from build123d import *

# Parameters (mm, degrees)
SKETCH1_R           = 11.025
BOSS_EXTRUDE1_DEPTH = 10
SKETCH3_R           = 11.025
SKETCH3_R_2         = 6
BOSS_EXTRUDE2_DEPTH = 4
FILLET1_R           = 4
FILLET2_R           = 1
CUT_EXTRUDE1_REACH  = 12
SKETCH4_R           = 2.6


with BuildPart() as part:
    # Sketch1 → Boss-Extrude1 (new body)
    with BuildSketch(Plane(origin=(0, 0, 0), x_dir=(1, 0, 0), z_dir=(0, 1, 0))):
        with BuildLine():
            Line((-40, -16.45412), (40, -16.45412))
            Line((40, -16.45412), (40, 0))
            Line((40, 0), (20.55, 0))
            ThreePointArc((20.55, 0), (0, 20.55), (-20.55, 0))
            Line((-20.55, 0), (-40, 0))
            Line((-40, 0), (-40, -16.45412))
        make_face()
        Circle(SKETCH1_R, mode=Mode.SUBTRACT)
    extrude(amount=BOSS_EXTRUDE1_DEPTH)

    # Sketch3 → Boss-Extrude2 (add)
    with BuildSketch(Plane.XZ):
        Circle(SKETCH3_R)
        Circle(SKETCH3_R_2, mode=Mode.SUBTRACT)
    extrude(amount=-BOSS_EXTRUDE2_DEPTH)

    # Fillet1
    fillet1_edges = [part.edges().sort_by_distance(p)[0] for p in [
        (-40, 5, 0),
        (-20.55, 5, 0),
        (20.55, 5, 0),
        (40, 5, 0),
    ]]
    fillet(fillet1_edges, radius=FILLET1_R)

    # Fillet2
    fillet2_edges = [part.edges().sort_by_distance(p)[0] for p in [
        (40, 10, 10.22706),
        (-11.025, 10, 0),
        (-6, 4, 0),
        (-40, 10, 10.22706),
        (-30.110971266, 10, 0),
        (30.110971266, 10, 0),
        (0, 10, -20.55),
        (38.828427125, 10, 1.171572875),
        (-38.828427125, 10, 1.171572875),
        (-21.634175603, 10, -0.949842246),
        (21.634175603, 10, -0.949842246),
    ]]
    fillet(fillet2_edges, radius=FILLET2_R)

    # Sketch4 → Cut-Extrude1 (cut, up to next)
    with BuildSketch(Plane.XZ, mode=Mode.PRIVATE) as cut_extrude1_sk1:
        with Locations((30, 8.22706)):
            Circle(SKETCH4_R)
    cut_extrude1_tool1 = extrude(cut_extrude1_sk1.sketch, amount=-CUT_EXTRUDE1_REACH, mode=Mode.PRIVATE) & part.part
    add(cut_extrude1_tool1.solids().sort_by_distance((30, 0, 8.22706))[0], mode=Mode.SUBTRACT)
    # Sketch4 → Cut-Extrude1 (cut, up to next)
    with BuildSketch(Plane.XZ, mode=Mode.PRIVATE) as cut_extrude1_sk2:
        with Locations((-29.996640074, 8.862024441)):
            Circle(SKETCH4_R)
    cut_extrude1_tool2 = extrude(cut_extrude1_sk2.sketch, amount=-CUT_EXTRUDE1_REACH, mode=Mode.PRIVATE) & part.part
    add(cut_extrude1_tool2.solids().sort_by_distance((-29.99664, 0, 8.862024))[0], mode=Mode.SUBTRACT)


solid = part.part
Geometry check sheet. Reference: the model listing, model coordinates, mm. A direction names the side the tool comes from. Give positions to 0.01 mm unless a question says otherwise; leave off trailing zeros. Loops run counter-clockwise (first coordinate to the right, second up) from the corner with the lowest first, then second, coordinate; pieces in that order, holes last. Notation, with made-up numbers: M -34,-1.75 L -6,-1.75 A16 ccw -6,19.25 Z; hole C 27,-30.5 d6. An arc over 180 degrees is marked long. Answer as a JSON object with one key per item and string values. Group by question number.
Item 1: Sectioned sample at A-A on x = 0. Record the boundary of the cut face in (y, z) (3 decimals).
Item 2: Gauge pin test, flat ends, axial feed: pin 1 (5 mm diameter, centred on y = 5, z = -11, fed in from -X); pin 2 (2.5 mm diameter, centred on x = 30.5, y = 4, fed in from -Z); pin 3 (1.5 mm diameter, centred on y = 3.5, z = -14.5, fed in from -X). Record the tip position at first contact, or that the pin passes through.
Item 3: Sectioned sample at C-C on x = 30. Record the boundary of the cut face in (y, z).
Item 4: Material ranges on L1, parallel to X at y = 5.25, z = 7; L2, parallel to X at y = 2.75, z = 8; L3, parallel to Z at x = -2, y = 2.25, recorded low to high.
Item 5: Sectioned sample at B-B on y = 7. Record the boundary of the cut face in (x, z) (3 decimals), plus the area to 3 significant figures.
Item 6: Access from +Z, -Z, +X, -X, +Y, -Y to the whole of each face (thin tool, end or side, straight path). Record for faces 4 (the flat face through (-0.2, 4, -7.2)), 5 (the flat face through (30, 4, 0)), 6 (the cylindrical face through (-27.595, 4.93, 7.866)), 7 (the flat face through (40, 4, 10)), 8 (the flat face through (-30, 4, 0)).
Item 7: Mould release check, pull along Z, two halves, no side actions. Record for faces 1 (the flat face through (-40, 4, 10)), 2 (the cylindrical face through (28.1, 4.9, 10)), 3 (the cylindrical face through (0.405, 4.437, -20.546)): pulls with the +Z half, pulls with the -Z half, needs draft (parallel to the pull), parting line crosses it, or undercut.
Findings below:
{
 "1": {"outline": "M 0,-20.55 L 9,-20.55 A1 ccw 10,-19.55 L 10,-12.025 A1 ccw 9,-11.025 L 4,-11.025 L 4,-7 A1 ccw 3,-6 L 0,-6 Z; M 0,6 L 3,6 A1 ccw 4,7 L 4,11.025 L 9,11.025 A1 ccw 10,12.025 L 10,16.454 L 0,16.454 Z"},
 "2": {"pin 1": "x = -18.71", "pin 2": "z = 0", "pin 3": "x = -15.27"},
 "3": {"outline": "M 0,0 L 9,0 A1 ccw 10,1 L 10,5.63 L 0,5.63 Z; M 0,10.83 L 10,10.83 L 10,16.45 L 0,16.45 Z"},
 "4": {"L1": "-40 to -31.81, -28.18 to -8.52, 8.52 to 27.71, 32.29 to 40", "L2": "-40 to -32.45, -27.54 to 27.41, 32.59 to 40", "L3": "-20.45 to -5.66, 5.66 to 16.45"},
 "5": {"outline": "M -40,4 A4 ccw -36,0 L -24.222,0 A4 cw -20.275,-3.348 A20.55 ccw 20.275,-3.348 A4 cw 24.222,0 L 36,0 A4 ccw 40,4 L 40,16.454 L -40,16.454 Z; hole C -29.997,8.862 d5.2; hole C 0,0 d22.05; hole C 30,8.227 d5.2", "area": "1,550 mm2"},
 "6": {"face 4": "+Y", "face 5": "-Z, +X, +Y, -Y", "face 6": "+Y, -Y", "face 7": "+Z, -Z, +X, +Y, -Y", "face 8": "-Z, -X, +Y, -Y"},
 "7": {"face 1": "needs draft", "face 2": "undercut", "face 3": "pulls with the -Z half"}
}
